Model file for the job. Use its own axes, mm. A direction names the side the tool comes from. Give positions to 0.01 mm unless a question says otherwise; leave off trailing zeros. Loops run counter-clockwise (first coordinate to the right, second up) from the corner with the lowest first, then second, coordinate; pieces in that order, holes last. Notation, with made-up numbers: M 1,-12 L 31,-12 A17 cw 31,3 Z; hole C 43,11 d11. An arc over 180 degrees is marked long. Answer in a Markdown table with one row per item.
```python
from build123d import *

# Parameters (mm, degrees)
ESQUISSE1_R        = 1
BOSS_EXTRU_1_DEPTH = 3


with BuildPart() as part:
    # Esquisse1 → Boss.-Extru.1 (new body)
    with BuildSketch(Plane(origin=(0, 0, 0), x_dir=(1, 0, 0), z_dir=(0, 1, 0))):
        with BuildLine():
            Line((-28, -30.8), (-25, -30.8))
            Line((-25, -30.8), (-25, -33.8))
            Line((-25, -33.8), (-17, -33.8))
            Line((-17, -33.8), (-17, -30.8))
            Line((-17, -30.8), (-11, -30.8))
            Line((-11, -30.8), (-11, -33.8))
            Line((-11, -33.8), (-3, -33.8))
            Line((-3, -33.8), (-3, -30.8))
            Line((-3, -30.8), (3, -30.8))
            Line((3, -30.8), (3, -33.8))
            Line((3, -33.8), (11, -33.8))
            Line((11, -33.8), (11, -30.8))
            Line((11, -30.8), (17, -30.8))
            Line((17, -30.8), (17, -33.8))
            Line((17, -33.8), (25, -33.8))
            Line((25, -33.8), (25, -30.8))
            Line((25, -30.8), (28, -30.8))
            Line((28, -30.8), (28, -3))
            ThreePointArc((28, -3), (27.121320344, -0.878679656), (25, 0))
            Line((25, 0), (-25, 0))
            ThreePointArc((-25, 0), (-27.121320344, -0.878679656), (-28, -3))
            Line((-28, -3), (-28, -30.8))
        make_face()
        with Locations(Location((-23.75, -4.25, 0), (0, 0, 270))):
            Circle(ESQUISSE1_R, mode=Mode.SUBTRACT)
        with Locations(Location((-23.75, -26.55, 0), (0, 0, 270))):
            Circle(ESQUISSE1_R, mode=Mode.SUBTRACT)
        with Locations(Location((23.75, -26.55, 0), (0, 0, 270))):
            Circle(ESQUISSE1_R, mode=Mode.SUBTRACT)
        with Locations(Location((23.75, -4.25, 0), (0, 0, 270))):
            Circle(ESQUISSE1_R, mode=Mode.SUBTRACT)
        with BuildLine():
            Line((-11.5, -11.55), (-8.5, -11.55))
            Line((-8.5, -11.55), (-8.5, -24.55))
            ThreePointArc((-8.5, -24.55), (-7.914213562, -25.964213562), (-6.5, -26.55))
            Line((-6.5, -26.55), (6.5, -26.55))
            ThreePointArc((6.5, -26.55), (7.914213562, -25.964213562), (8.5, -24.55))
            Line((8.5, -24.55), (8.5, -11.55))
            Line((8.5, -11.55), (11.5, -11.55))
            Line((11.5, -11.55), (11.5, -4.25))
            Line((11.5, -4.25), (-11.5, -4.25))
            Line((-11.5, -4.25), (-11.5, -11.55))
        make_face(mode=Mode.SUBTRACT)
    extrude(amount=BOSS_EXTRU_1_DEPTH)


solid = part.part
```
Q1. Saw through at C-C (y = 2.3). Give the number of separate pieces and of enclosed holes in the cut face, and give its area (3 significant figures).
Reported:
| item | result |
|---|---|
| separate pieces | 1 |
| enclosed holes | 5 |
| area | 1,380 mm² |
Q2. Saw through at B-B (x = 23.75). Give the cut face in (y, z), and give its area (3 significant figures).
Reported:
| item | result |
|---|---|
| outline | M 0,0 L 3,0 L 3,3.25 L 0,3.25 Z; M 0,5.25 L 3,5.25 L 3,25.55 L 0,25.55 Z; M 0,27.55 L 3,27.55 L 3,33.8 L 0,33.8 Z |
| area | 89.4 mm² |
Q3. Probe probe 1 along X at (y, z) = (1.9, 8); probe 2 along Z at (x, y) = (-9, 0.75); probe 3 along X at (y, z) = (1.9, 24.5). List the from-to ranges inside material, lowest first.
Reported:
| item | result |
|---|---|
| probe 1 | -28 to -11.5, 11.5 to 28 |
| probe 2 | 0 to 4.25, 11.55 to 33.8 |
| probe 3 | -28 to -8.5, 8.5 to 28 |
Q4. Drop flat-ended pins along their axis: pin 1 (1.5 mm diameter, centred on y = 1.5, z = 32.5, fed in from -X); pin 2 (0.9 mm diameter, centred on x = 14.5, y = 1.5, fed in from +Z). Give the stop position or say it passes through.
Reported:
| item | result |
|---|---|
| pin 1 | x = -25 |
| pin 2 | z = 30.8 |
Q5. Saw through at A-A (z = 24). Give the cut face in (x, y).
Reported:
| item | result |
|---|---|
| outline | M -28,0 L -8.5,0 L -8.5,3 L -28,3 Z; M 8.5,0 L 28,0 L 28,3 L 8.5,3 Z |
Q6. Mould opens along Z. For faces 1 (the face through (8.5, 1, 18)), 2 (the face through (25, 1, 32)), 3 (the face through (21, 1, 33.8)) say: released by +Z, released by -Z, zero draft, split by the parting line, or undercut.
Reported:
| item | result |
|---|---|
| face 1 | undercut |
| face 2 | zero draft |
| face 3 | released by +Z |
Q7. 3-axis set-ups, long thin cutter, end or side, ignore diameter. For faces 4 (the face through (-10, 1, 11.55)), 5 (the face through (26, 1, 30.8)), 6 (the face through (-17, 1, 32)): which of +Z, -Z, +X, -X, +Y, -Y reach the whole face in a straight line?
Reported:
| item | result |
|---|---|
| face 4 | +Y, -Y |
| face 5 | +Z, +X, +Y, -Y |
| face 6 | +Z, +Y, -Y |
